from build123d import *

# Parameters (mm, degrees)
SKETCH_1_W                        = 199
SKETCH_1_H                        = 149
SKETCH_1_R                        = 3
SKETCH_1_W_2                      = 46
SKETCH_1_H_2                      = 94
SM_BASE_FLANGE_1_DEPTH            = 0.8
SM_EDGE_FLANGE_1_STRIP_W          = 4.2
SM_EDGE_FLANGE_1_STRIP_H          = 0.8
SM_EDGE_FLANGE_1_STRIP_CUT_DEPTH  = 59
SM_EDGE_FLANGE_1_RELIEF_W         = 5
SM_EDGE_FLANGE_1_RELIEF_H         = 0.8
SM_EDGE_FLANGE_1_RELIEF_CUT_DEPTH = 0.8
SM_EDGE_FLANGE_1_DEPTH            = 59
SM_EDGE_FLANGE_3_STRIP_W          = 4.2
SM_EDGE_FLANGE_3_STRIP_H          = 0.8
SM_EDGE_FLANGE_3_STRIP_CUT_DEPTH  = 139
SM_EDGE_FLANGE_3_RELIEF_W         = 5
SM_EDGE_FLANGE_3_RELIEF_H         = 0.8
SM_EDGE_FLANGE_3_RELIEF_CUT_DEPTH = 0.8
SM_EDGE_FLANGE_3_DEPTH            = 139
SM_EDGE_FLANGE_3_FLAT_DEPTH       = 0.8
SM_EDGE_FLANGE_4_STRIP_W          = 4.2
SM_EDGE_FLANGE_4_STRIP_H          = 0.8
SM_EDGE_FLANGE_4_STRIP_CUT_DEPTH  = 139
SM_EDGE_FLANGE_4_RELIEF_W         = 5
SM_EDGE_FLANGE_4_RELIEF_H         = 0.8
SM_EDGE_FLANGE_4_RELIEF_CUT_DEPTH = 0.8
SM_EDGE_FLANGE_4_DEPTH            = 139
SM_EDGE_FLANGE_4_FLAT_DEPTH       = 0.8
SM_EDGE_FLANGE_5_STRIP_W          = 4.2
SM_EDGE_FLANGE_5_STRIP_H          = 0.8
SM_EDGE_FLANGE_5_STRIP_CUT_DEPTH  = 149
SM_EDGE_FLANGE_5_DEPTH            = 149
SKETCH_21_R                       = 4
CUT_EXTRUDE_1_DEPTH               = 214.427388121


# Sheet-metal steps are written as plain solids
with BuildPart() as part:
    # Sketch 1 → 基体-法兰1 (new body)
    with BuildSketch(Plane.XY):
        Rectangle(SKETCH_1_W, SKETCH_1_H)
        with Locations((-89.5, 64.5)):
            Circle(SKETCH_1_R, mode=Mode.SUBTRACT)
        with Locations((-89.5, -64.5)):
            Circle(SKETCH_1_R, mode=Mode.SUBTRACT)
        with Locations((58.5, 0)):
            Rectangle(SKETCH_1_W_2, SKETCH_1_H_2, mode=Mode.SUBTRACT)
    extrude(amount=-SM_BASE_FLANGE_1_DEPTH)

    # 边线-法兰1 strip (across the edge) → 边线-法兰1 strip cut (cut)
    with BuildSketch(Plane(origin=(-99.5, -29.5, -0.8), x_dir=(1, 0, 0), z_dir=(0, 1, 0))):
        with Locations((-0.8, -0.4)):
            Rectangle(SM_EDGE_FLANGE_1_STRIP_W, SM_EDGE_FLANGE_1_STRIP_H)
    extrude(amount=SM_EDGE_FLANGE_1_STRIP_CUT_DEPTH, mode=Mode.SUBTRACT)

    # 边线-法兰1 relief (on the sheet) → 边线-法兰1 relief cut (cut)
    with BuildSketch(Plane(origin=(-98.2, -29.5, -0.8), x_dir=(1, 0, 0), z_dir=(0, 0, -1))):
        with Locations((-1.7, 0.4)):
            Rectangle(SM_EDGE_FLANGE_1_RELIEF_W, SM_EDGE_FLANGE_1_RELIEF_H)
        with Locations((-1.7, -59.4)):
            Rectangle(SM_EDGE_FLANGE_1_RELIEF_W, SM_EDGE_FLANGE_1_RELIEF_H)
    extrude(amount=-SM_EDGE_FLANGE_1_RELIEF_CUT_DEPTH, mode=Mode.SUBTRACT)

    # 边线-法兰1 section (across the edge) → 边线-法兰1 (add)
    with BuildSketch(Plane(origin=(-99.5, -29.5, -0.8), x_dir=(1, 0, 0), z_dir=(0, 1, 0))):
        with BuildLine():
            Line((0, 0.5), (0, 19.2))
            Line((0, 19.2), (0.8, 19.2))
            Line((0.8, 19.2), (0.8, 0.5))
            ThreePointArc((0.8, 0.5), (0.946446609, 0.146446609), (1.3, 0))
            Line((1.3, 0), (1.3, -0.8))
            ThreePointArc((1.3, -0.8), (0.380761184, -0.419238816), (0, 0.5))
        make_face()
    extrude(amount=SM_EDGE_FLANGE_1_DEPTH)

    # 边线-法兰3 strip (across the edge) → 边线-法兰3 strip cut (cut)
    with BuildSketch(Plane(origin=(89.5, -74.5, -0.8), x_dir=(0, 1, 0), z_dir=(-1, 0, 0))):
        with Locations((-0.8, -0.4)):
            Rectangle(SM_EDGE_FLANGE_3_STRIP_W, SM_EDGE_FLANGE_3_STRIP_H)
    extrude(amount=SM_EDGE_FLANGE_3_STRIP_CUT_DEPTH, mode=Mode.SUBTRACT)

    # 边线-法兰3 relief (on the sheet) → 边线-法兰3 relief cut (cut)
    with BuildSketch(Plane(origin=(89.5, -73.2, -0.8), x_dir=(0, 1, 0), z_dir=(0, 0, -1))):
        with Locations((-1.7, 0.4)):
            Rectangle(SM_EDGE_FLANGE_3_RELIEF_W, SM_EDGE_FLANGE_3_RELIEF_H)
        with Locations((-1.7, -139.4)):
            Rectangle(SM_EDGE_FLANGE_3_RELIEF_W, SM_EDGE_FLANGE_3_RELIEF_H)
    extrude(amount=-SM_EDGE_FLANGE_3_RELIEF_CUT_DEPTH, mode=Mode.SUBTRACT)

    # 边线-法兰3 bend section (across the edge) → 边线-法兰3 (add)
    with BuildSketch(Plane(origin=(89.5, -74.5, -0.8), x_dir=(0, 1, 0), z_dir=(-1, 0, 0))):
        with BuildLine():
            Line((0, 0.5), (0.8, 0.5))
            ThreePointArc((0.8, 0.5), (0.946446609, 0.146446609), (1.3, 0))
            Line((1.3, 0), (1.3, -0.8))
            ThreePointArc((1.3, -0.8), (0.380761184, -0.419238816), (0, 0.5))
        make_face()
    extrude(amount=SM_EDGE_FLANGE_3_DEPTH)

    # 边线-法兰3 profile (on flange) → 边线-法兰3 flat (add)
    with BuildSketch(Plane(origin=(0, -74.5, -0.8), x_dir=(-1, 0, 0), z_dir=(0, -1, 0))):
        Polygon((49.5, 0.5), (49.5, 19.2), (15.5, 19.2), (15.5, 4.2), (-29.5, 4.2), (-29.5, 19.2), (-89.5, 19.2), (-89.5, 0.5), align=None)
    extrude(amount=-SM_EDGE_FLANGE_3_FLAT_DEPTH)

    # 边线-法兰4 strip (across the edge) → 边线-法兰4 strip cut (cut)
    with BuildSketch(Plane(origin=(-49.5, 74.5, -0.8), x_dir=(0, -1, 0), z_dir=(1, 0, 0))):
        with Locations((-0.8, -0.4)):
            Rectangle(SM_EDGE_FLANGE_4_STRIP_W, SM_EDGE_FLANGE_4_STRIP_H)
    extrude(amount=SM_EDGE_FLANGE_4_STRIP_CUT_DEPTH, mode=Mode.SUBTRACT)

    # 边线-法兰4 relief (on the sheet) → 边线-法兰4 relief cut (cut)
    with BuildSketch(Plane(origin=(-49.5, 73.2, -0.8), x_dir=(0, -1, 0), z_dir=(0, 0, -1))):
        with Locations((-1.7, 0.4)):
            Rectangle(SM_EDGE_FLANGE_4_RELIEF_W, SM_EDGE_FLANGE_4_RELIEF_H)
        with Locations((-1.7, -139.4)):
            Rectangle(SM_EDGE_FLANGE_4_RELIEF_W, SM_EDGE_FLANGE_4_RELIEF_H)
    extrude(amount=-SM_EDGE_FLANGE_4_RELIEF_CUT_DEPTH, mode=Mode.SUBTRACT)

    # 边线-法兰4 bend section (across the edge) → 边线-法兰4 (add)
    with BuildSketch(Plane(origin=(-49.5, 74.5, -0.8), x_dir=(0, -1, 0), z_dir=(1, 0, 0))):
        with BuildLine():
            Line((0, 0.5), (0.8, 0.5))
            ThreePointArc((0.8, 0.5), (0.946446609, 0.146446609), (1.3, 0))
            Line((1.3, 0), (1.3, -0.8))
            ThreePointArc((1.3, -0.8), (0.380761184, -0.419238816), (0, 0.5))
        make_face()
    extrude(amount=SM_EDGE_FLANGE_4_DEPTH)

    # 边线-法兰4 profile (on flange) → 边线-法兰4 flat (add)
    with BuildSketch(Plane(origin=(0, 74.5, -0.8), x_dir=(1, 0, 0), z_dir=(0, 1, 0))):
        Polygon((89.5, 0.5), (89.5, 19.2), (29.5, 19.2), (29.5, 4.2), (-15.5, 4.2), (-15.5, 19.2), (-49.5, 19.2), (-49.5, 0.5), align=None)
    extrude(amount=-SM_EDGE_FLANGE_4_FLAT_DEPTH)

    # 边线-法兰5 strip (across the edge) → 边线-法兰5 strip cut (cut)
    with BuildSketch(Plane(origin=(99.5, 74.5, -0.8), x_dir=(-1, 0, 0), z_dir=(0, -1, 0))):
        with Locations((-0.8, -0.4)):
            Rectangle(SM_EDGE_FLANGE_5_STRIP_W, SM_EDGE_FLANGE_5_STRIP_H)
    extrude(amount=SM_EDGE_FLANGE_5_STRIP_CUT_DEPTH, mode=Mode.SUBTRACT)

    # 边线-法兰5 section (across the edge) → 边线-法兰5 (add)
    with BuildSketch(Plane(origin=(99.5, 74.5, -0.8), x_dir=(-1, 0, 0), z_dir=(0, -1, 0))):
        with BuildLine():
            Line((0, 0.5), (0, 19.2))
            Line((0, 19.2), (0.8, 19.2))
            Line((0.8, 19.2), (0.8, 0.5))
            ThreePointArc((0.8, 0.5), (0.946446609, 0.146446609), (1.3, 0))
            Line((1.3, 0), (1.3, -0.8))
            ThreePointArc((1.3, -0.8), (0.380761184, -0.419238816), (0, 0.5))
        make_face()
    extrude(amount=SM_EDGE_FLANGE_5_DEPTH)

    # 草图21 → 切除-拉伸1 (cut, through all)
    with BuildSketch(Plane(origin=(99.5, 0, 0), x_dir=(0, 0, -1), z_dir=(1, 0, 0))):
        with Locations((10, -39)):
            Circle(SKETCH_21_R)
        with Locations((10, 39)):
            Circle(SKETCH_21_R)
    extrude(amount=-CUT_EXTRUDE_1_DEPTH, mode=Mode.SUBTRACT)


solid = part.part
Read the model definition and answer for the solid it produces. Units are mm, in the model's axes. A direction names the side the tool comes from. Coordinates: 2 decimals unless noted, no trailing zeros. Loops run counter-clockwise (first coordinate to the right, second up) from the corner with the lowest first, then second, coordinate; pieces in that order, holes last. Notation, with made-up numbers: (-34.75, -26.75) - (-5.75, -26.75) arc R5 ccw to (-5.75, -20.75) - close; hole circle Ø2 at (79.5, -6.75). An arc over 180 degrees is marked (long way). Answer in a Markdown table with one row per item.
Q1. The mould has two halves that part along Y. Classify faces 1 (the cylindrical face through (99.106, -35.034, -9.479)), 2 (the flat face through (-2, 1, 0)), 3 (the flat face through (99, 74.5, -7)): pulls with the +Y half, pulls with the -Y half, needs draft (parallel to the pull), parting line crosses it, or undercut.
Here are the results:
| item | result |
|---|---|
| face 1 | undercut |
| face 2 | needs draft |
| face 3 | pulls with the +Y half |
Q2. Find section C-C on x = -89.5. Write down the section's boundary in (y, z).
Here are the results:
| item | result |
|---|---|
| outline | (-74.5, -0.8) - (-67.5, -0.8) - (-67.5, 0) - (-74.5, 0) - close; (-61.5, -0.8) - (61.5, -0.8) - (61.5, 0) - (-61.5, 0) - close; (67.5, -0.8) - (74.5, -0.8) - (74.5, 0) - (67.5, 0) - close |
Q3. Find section D-D on y = 64.5. Write down the section's boundary in (x, z), plus the area to 3 significant figures.
Here are the results:
| item | result |
|---|---|
| outline | (-99.5, -0.8) - (-92.5, -0.8) - (-92.5, 0) - (-99.5, 0) - close; (-86.5, -0.8) - (98.2, -0.8) arc R0.5 cw to (98.7, -1.3) - (98.7, -20) - (99.5, -20) - (99.5, -1.3) arc R1.3 ccw to (98.2, 0) - (-86.5, 0) - close |
| area | 169 mm^2 |
Q4. Given P1, Ø4, axis at x = -45.5, y = 29.5, coming from the -Z side; P2, Ø0.6, axis at y = -74, z = -12.5, coming from the -X side; P3, Ø0.9, axis at x = -50, z = -0.5, coming from the +Y side; P4, Ø1.7, axis at x = -99, z = -6.5, coming from the +Y side, each flat-ended and moving along its own axis, determine where each tip first touches the part or whether it passes through.
Here are the results:
| item | result |
|---|---|
| P1 | stops at z = -0.8 |
| P2 | stops at x = -49.5 |
| P3 | stops at y = 74.5 |
| P4 | stops at y = 29.5 |
Q5. For faces 4 (the flat face through (-2, 1, -0.8)), 5 (the flat face through (-98.7, 0, -11)), 6 (the flat face through (21, -73.7, -4.5)), determine the directions among +Z, -Z, +X, -X, +Y, -Y from which every point of the face is accessible in a straight line to the end or side of a thin tool.
Here are the results:
| item | result |
|---|---|
| face 4 | -Z |
| face 5 | -Z, +Y, -Y |
| face 6 | -Z, -X |
Q6. Straight lines are drawn through the part: line 1 along Y through (x, z) = (99, -10); line 2 along Y through (x, z) = (48, -3.5); line 3 along X through (y, z) = (23.5, -10.5). For each, find the intervals that lie inside material, in ascending order. Write a range as [from, to].
Here are the results:
| item | result |
|---|---|
| line 1 | y = [-74.5, -43], [-35, 35], [43, 74.5] |
| line 2 | y = [-74.5, -73.7], [73.7, 74.5] |
| line 3 | x = [-99.5, -98.7], [98.7, 99.5] |
Q7. Find section A-A on y = -39. Write down the section's boundary in (x, z).
Here are the results:
| item | result |
|---|---|
| outline | (-99.5, -0.8) - (35.5, -0.8) - (35.5, 0) - (-99.5, 0) - close; (81.5, -0.8) - (98.2, -0.8) arc R0.5 cw to (98.7, -1.3) - (98.7, -6) - (99.5, -6) - (99.5, -1.3) arc R1.3 ccw to (98.2, 0) - (81.5, 0) - close; (98.7, -20) - (99.5, -20) - (99.5, -14) - (98.7, -14) - close |
Q8. Find section B-B on z = -10. Count the separate pieces of the cut face and the enclosed holes in it, plus the area to 3 significant figures.
Here are the results:
| item | result |
|---|---|
| separate pieces | 8 |
| enclosed holes | 0 |
| area | 304 mm^2 |
